The model under review builds one solid part; all positions refer to its coordinate system, in mm. A direction names the side the tool comes from. Coordinates: 2 decimals unless noted, no trailing zeros. Order: outer loops, then holes, each group sorted by start corner. A loop starts at its lowest first (then second) coordinate and runs counter-clockwise, first axis right, second up.
Solid Edge part; units mm, degrees
sketch "Sketch1" plane through (0, 0, 0) normal (0, 0, 1) x (1, 0, 0)
  spline S0 degree 3 poles (-69.5242, 19.4932) (-23.3267, 12.9257) (22.6888, 12.9752) (68.6585, 19.674) knots 0 0 0 0 1 1 1 1
  spline S1 degree 3 poles (-69.54, -19.6556) (-23.1773, -15.4302) (23.2615, -15.4924) (69.7765, -19.8423) knots 0 0 0 0 1 1 1 1
  arc A0 (-69.54, -19.6556) -> (-69.5242, 19.4932) centre (-75.1666, -0.0789) cw
  arc A1 (68.6585, 19.674) -> (69.7765, -19.8423) centre (75.0403, 0.0806) cw
extrude "Protrusion1" add sketch "Sketch1" along normal blind 3
sketch "Sketch2" plane through (0.0555, 0.0806, 3) normal (0, 0, 1) x (1, 0, 0)
  circle A0 centre (83.5848, 0) radius 1
  circle A1 centre (55.6848, 0) radius 1
  line L0 (-58.5721, -6.5095) -> (-58.5721, 6.1905)
  line L1 (-58.5721, 6.1905) -> (-81.1721, 6.1905)
  line L2 (-81.1721, 6.1905) -> (-81.1721, -6.5095)
  line L3 (-81.1721, -6.5095) -> (-58.5721, -6.5095)
  circle A2 centre (-83.8221, -0.1595) radius 1
  circle A3 centre (-55.9221, -0.1595) radius 1
  line L4 (58.3348, 6.35) -> (58.3348, -6.35)
  line L5 (58.3348, -6.35) -> (80.9348, -6.35)
  line L6 (80.9348, -6.35) -> (80.9348, 6.35)
  line L7 (80.9348, 6.35) -> (58.3348, 6.35)
  dimension "D1" = 58.3348
  dimension "D2" = 58.3348
  dimension "D3" = 58.3348
extrude "ExtrudedCutout_1" cut sketch "Sketch2" against normal blind 484.752
sketch "Sketch3" plane through (0.0555, 0.0806, 3) normal (0, 0, 1) x (1, 0, 0)
  line L0 (29.6848, 27.4896) -> (-99.1539, 27.4896)
  line L1 (-99.1539, 27.4896) -> (-99.1539, -25.8213)
  line L2 (-99.1539, -25.8213) -> (29.6848, -25.8213)
  line L3 (29.6848, -25.8213) -> (29.6848, 27.4896)
extrude "ExtrudedCutout_2" cut sketch "Sketch3" against normal blind 169.5138
sketch "Sketch4" plane through (0, 0, 0) normal (0, 0, 1) x (1, 0, 0)
  line L0 (29.7403, -17.1563) -> (29.7403, 15.5915)
  spline S0 degree 3 poles (29.7403, 15.5915) (42.2697, 16.3768) (55.2702, 17.7412) (68.6585, 19.674) knots 0 0 0 0 1 1 1 1
  spline S1 degree 3 poles (29.7403, -17.1563) (34.3353, -17.3622) (40.0841, -17.6253) (48.6781, -18.1532) (57.9287, -18.805) (64.4454, -19.3301) (69.7765, -19.8423) knots 0 0 0 0 0.312805 0.467988 0.637686 1 1 1 1
  arc A0 (68.6585, 19.674) -> (69.7765, -19.8423) centre (75.0403, 0.0806) cw
  line L1 (58.3903, -6.2694) -> (58.3903, 6.4306)
  line L2 (58.3903, 6.4306) -> (80.9903, 6.4306)
  line L3 (80.9903, 6.4306) -> (80.9903, -6.2694)
  line L4 (80.9903, -6.2694) -> (58.3903, -6.2694)
  circle A1 centre (55.7403, 0.0806) radius 1
  circle A2 centre (83.6403, 0.0806) radius 1
  line L5 (29.7403, -17.1563) -> (29.7403, 15.5915)
  spline S2 degree 3 poles (29.7403, 15.5915) (17.2109, 16.3768) (4.2104, 17.7412) (-9.1779, 19.674) knots 0 0 0 0 1 1 1 1
  arc A3 (-9.1779, 19.674) -> (-10.2959, -19.8423) centre (-15.5597, 0.0806) ccw
  spline S3 degree 3 poles (29.7403, -17.1563) (25.1453, -17.3622) (19.3965, -17.6253) (10.8024, -18.1532) (1.5519, -18.805) (-4.9648, -19.3301) (-10.2959, -19.8423) knots 0 0 0 0 0.312805 0.467988 0.637686 1 1 1 1
  line L6 (1.0903, -6.2694) -> (1.0903, 6.4306)
  line L7 (1.0903, 6.4306) -> (-21.5097, 6.4306)
  line L8 (-21.5097, 6.4306) -> (-21.5097, -6.2694)
  line L9 (-21.5097, -6.2694) -> (1.0903, -6.2694)
  circle A4 centre (3.7403, 0.0806) radius 1
  circle A5 centre (-24.1597, 0.0806) radius 1
extrude "ExtrudedProtrusion_2" add sketch "Sketch4" against normal blind 3
sketch "Sketch5" plane through (-3.213, 0.0806, 0) normal (0, 0, 1) x (0, 1, 0)
  line L0 (25.6992, -32.9533) -> (-24.0131, -32.9533)
  line L1 (-24.0131, -32.9533) -> (-24.0131, 35.3247)
  line L2 (-24.0131, 35.3247) -> (25.6992, 35.3247)
  line L3 (25.6992, 35.3247) -> (25.6992, -32.9533)
extrude "ExtrudedCutout_3" cut sketch "Sketch5" against normal blind 310.7547
sketch "Sketch6" plane through (69.6903, 6.4306, 0) normal (0, -1, 0) x (1, 0, 0)
  line L0 (-39.95, 3) -> (25.9565, 3)
  line L1 (25.9565, 3) -> (25.9565, 0)
  line L2 (25.9565, 0) -> (-39.95, 0)
  line L3 (-39.95, 0) -> (-39.95, 3)
extrude "ExtrudedCutout_4" cut sketch "Sketch6" against normal blind 369.6121
sketch "Sketch7" plane through (69.6903, -6.2694, 0) normal (0, 1, 0) x (1, 0, 0)
  line L0 (-39.95, -0.4111) -> (-39.95, -3)
  line L1 (-39.95, -3) -> (25.7218, -3)
  line L2 (25.7218, -3) -> (25.9565, 0)
  line L3 (25.9565, 0) -> (-39.95, -0.4111)
extrude "ExtrudedCutout_5" cut sketch "Sketch7" against normal blind 176.465
sketch "Sketch8" plane through (29.7403, -0.7635, 0) normal (-1, 0, 0) x (0, -1, 0)
  line L0 (20.933, 0) -> (-7.194, 0)
  line L1 (-7.194, 0) -> (-7.194, 4.1468)
  line L2 (-7.194, 4.1468) -> (20.933, 4.1468)
  line L3 (20.933, 4.1468) -> (20.933, 0)
extrude "ExtrudedCutout_6" cut sketch "Sketch8" against normal blind 228.3963
sketch "Sketch9" plane through (0, 0, 0) normal (0, 0, 1) x (1, 0, 0)
  line L0 (-21.5097, -6.2694) -> (-21.5097, 6.4306)
  line L1 (-21.5097, 6.4306) -> (1.0903, 6.4306)
  line L2 (1.0903, -6.2694) -> (1.0903, 6.4306)
  line L3 (1.0903, -6.2694) -> (-21.5097, -6.2694)
  circle A0 centre (3.7403, 0.0806) radius 1
  circle A1 centre (-24.1597, 0.0806) radius 1
  spline S0 degree 3 poles (29.7403, 15.5915) (17.2977, 16.3681) (4.325, 17.7289) (-9.1779, 19.674) knots 0 0 0 0 1 1 1 1
  arc A2 (-9.1779, 19.674) -> (-10.2959, -19.8423) centre (-15.5597, 0.0806) ccw
  spline S1 degree 3 poles (29.7403, -17.1563) (17.4202, -17.6536) (4.1171, -18.5003) (-10.2959, -19.8423) knots 0 0 0 0 1 1 1 1
  line L4 (29.7403, -17.1563) -> (29.7403, 15.5915)
extrude "ExtrudedProtrusion_3" add sketch "Sketch9" against normal blind 3
(1) Consider section C-C (y = -12). Give the boundary of the cut face in (x, z), then the cut area to 3 significant figures.
(2) Consider section B-B (z = -0.6). Give the number of separate pieces and of enclosed holes in the cut face, then the cut area to 3 significant figures.
(3) Tool access review of faces 1 (the face through (80.99, 0, -1)), 2 (the face through (29, 0, 0)): name each direction out of +Z, -Z, +X, -X, +Y, -Y from which nothing blocks a thin tool from reaching the whole face with its end or side.
(4) Wall thickness on line 1 (Y direction, x = -16.5, z = -1.4); line 2 (X direction, y = -1.5, z = -2.3); line 3 (Y direction, x = -21, z = -1.1): over which ranges is each line inside the solid? List them lowest first.
(5) The part is to be moulded in two halves that separate along X. For faces 3 (the face through (-10, -6.269, -1)), 4 (the face through (29, 0, -3)), say which applies: +X half, -X half, draft (parallel to the pull), parting line (faces both ways), or undercut.
(6) Insertion check: pin 1 Ø3 at (x, y) = (-24.16, 0.08) entering from -Z; pin 2 Ø1.2 at (x, y) = (55.74, 0.08) entering from +Z; pin 3 Ø1.5 at (x, z) = (72, -1.5) entering from +Y; pin 4 Ø1.5 at (y, z) = (1, -1) entering from +X. Each pin has a flat end and moves straight along its axis. Give the tip position at first contact, or say it passes through.
(7) Consider section A-A (y = 2.5). Give the boundary of the cut face in (x, z).
Findings:
1. outline: (-32.25, -3) - (91.73, -3) - (91.73, 0) - (-32.25, 0) - close
1. area: 372 mm2
2. separate pieces: 1
2. enclosed holes: 6
2. area: 4,040 mm2
3. face 1: +Z, -Z
3. face 2: +Z, +X, -X, +Y, -Y
4. line 1: y = -20.5 to -6.27, 6.43 to 20.67
4. line 2: x = -36.11 to -21.51, 1.09 to 58.39, 80.99 to 95.59
4. line 3: y = -19.79 to -6.27, 6.43 to 19.96
5. face 3: undercut
5. face 4: draft
6. pin 1: stops at z = -3
6. pin 2: passes through
6. pin 3: stops at y = 20.56
6. pin 4: stops at x = 95.65
7. outline: (-36.02, -3) - (-21.51, -3) - (-21.51, 0) - (-36.02, 0) - close; (1.09, -3) - (58.39, -3) - (58.39, 0) - (1.09, 0) - close; (80.99, -3) - (95.5, -3) - (95.5, 0) - (80.99, 0) - close
